The listing builds one solid part. Answer for the finished solid, in the listing's coordinates (mm). Face numbers are marked on the shaded views. A direction names the side the tool comes from. Round coordinates to 2 decimals unless told otherwise and drop trailing zeros. Loops run counter-clockwise (first coordinate to the right, second up) from the corner with the lowest first, then second, coordinate; pieces in that order, holes last. Notation, with made-up numbers: (69, -13) -> (120, -13) arc R24 cw to (120, -2) -> close; hole circle Ø2 at (8, 17). An arc over 180 degrees is marked (long way). Write each question's results on one line, items separated by ' | '. Start each with the question number.
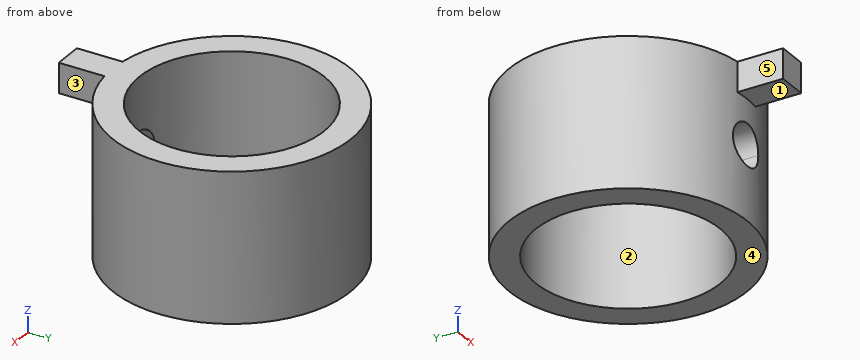
from build123d import *

# Parameters (mm, degrees)
F0_R     = 10.16
F1_DEPTH = 12.7
F3_DEPTH = 13.97
F5_DEPTH = 10.16
F7_D     = 15.748


with BuildPart() as f1:
    # F0 (on Top) → F1 (new body)
    with BuildSketch(Plane.XY):
        Circle(F0_R)
    extrude(amount=F1_DEPTH)

    # F2 (on Front) → F3 (join)
    with BuildSketch(Plane.XZ):
        Polygon((-1.27, 12.7), (-1.27, 10.16), (0, 10.16), (1.27, 10.16), (1.27, 12.7), align=None)
    extrude(amount=F3_DEPTH)

    # F4 (on Front) → F5 (cut, through all)
    with BuildSketch(Plane.XZ):
        with BuildLine():
            ThreePointArc((0, 4.572), (1.257236, 5.092764), (1.778, 6.35))
            ThreePointArc((1.778, 6.35), (-1.257236, 7.607236), (0, 4.572))
        make_face()
    extrude(amount=F5_DEPTH, mode=Mode.SUBTRACT)

    # F7 (through all)
    with Locations(Plane(origin=(0, 0, 0), x_dir=(1, 0, 0), z_dir=(0, 0, -1))):
        with Locations((0, 0)):
            Hole(F7_D / 2)


solid = f1.part
Item 1: Straight lines are drawn through the part: L1, parallel to Z at x = 0, y = -9.05; L2, parallel to Y at x = 0, z = 4.25; L3, parallel to Y at x = 0, z = 5.25. For each, find the intervals that lie inside material, in ascending order. Write a range as [from, to].
Item 2: The part is cut by section B-B, the plane z = 11. Give the vertices of the cut face in (x, y).
Item 3: The part is cut by section A-A, the plane y = 0. Give the vertices of the cut face in (x, z).
Item 4: The part is cut by section C-C, the plane x = 4. Give the vertices of the cut face in (y, z).
Item 5: The part is cut by section D-D, the plane z = 7.5. Give the vertices of the cut face in (x, y), plus the area to 3 significant figures.
Item 6: Each of these flat-tipped pins is pushed along its axis until it touches: pin 1 Ø1.3 at (x, y) = (0, -11.5) entering from -Z; pin 2 Ø5 at (x, y) = (1, 4) entering from +Z; pin 3 Ø4 at (x, z) = (3.5, 7) entering from -Y; pin 4 Ø3 at (x, z) = (-5, 9.5) entering from +Y. Where does it stop, or does it pass through?
Item 7: Determine the mould class of the marked faces 1, 2 and 3 for opening direction X: +X half, -X half, draft (parallel to the pull), parting line (faces both ways), or undercut.
Item 8: For the marked faces 4 and 5, determine the directions among +Z, -Z, +X, -X, +Y, -Y from which every point of the face is accessible in a straight line to the end or side of a thin tool.
Report:
1) L1: z = [0, 4.57], [8.13, 12.7] | L2: y = [-10.16, -7.87], [7.87, 10.16] | L3: y = [7.87, 10.16]
2) outline: (-1.27, -13.97) -> (1.27, -13.97) -> (1.27, -10.08) arc R10.16 ccw (long way) to (-1.27, -10.08) -> close; hole circle Ø15.75 at (0, 0)
3) outline: (-10.16, 0) -> (-7.87, 0) -> (-7.87, 12.7) -> (-10.16, 12.7) -> close; (7.87, 0) -> (10.16, 0) -> (10.16, 12.7) -> (7.87, 12.7) -> close
4) outline: (-9.34, 0) -> (-6.78, 0) -> (-6.78, 12.7) -> (-9.34, 12.7) -> close; (6.78, 0) -> (9.34, 0) -> (9.34, 12.7) -> (6.78, 12.7) -> close
5) outline: (-1.36, -10.07) -> (-1.36, -7.76) arc R7.87 cw (long way) to (1.36, -7.76) -> (1.36, -10.07) arc R10.16 ccw (long way) to start | area: 123 mm2
6) pin 1: stops at z = 10.16 | pin 2: passes through | pin 3: stops at y = -10.05 | pin 4: stops at y = 9.54
7) face 1: draft | face 2: undercut | face 3: +X half
8) face 4: -Z, +X, -X, +Y, -Y | face 5: +Z, -Z, -X, -Y
